Print and shaded views of the part. All mm, measured from the part's lowest x, y and z. A direction names the side the tool comes from. Round coordinates to 2 decimals unless told otherwise and drop trailing zeros. Order: outer loops, then holes, each group sorted by start corner. A loop starts at its lowest first (then second) coordinate and runs counter-clockwise, first axis right, second up. Notation, with made-up numbers: (-3, 11.5) - (6, 11.5) arc R14 cw to (6, 22.5) - close; hole circle Ø9 at (-10, 20.25). An arc over 180 degrees is marked (long way). Write item = value, one per line.
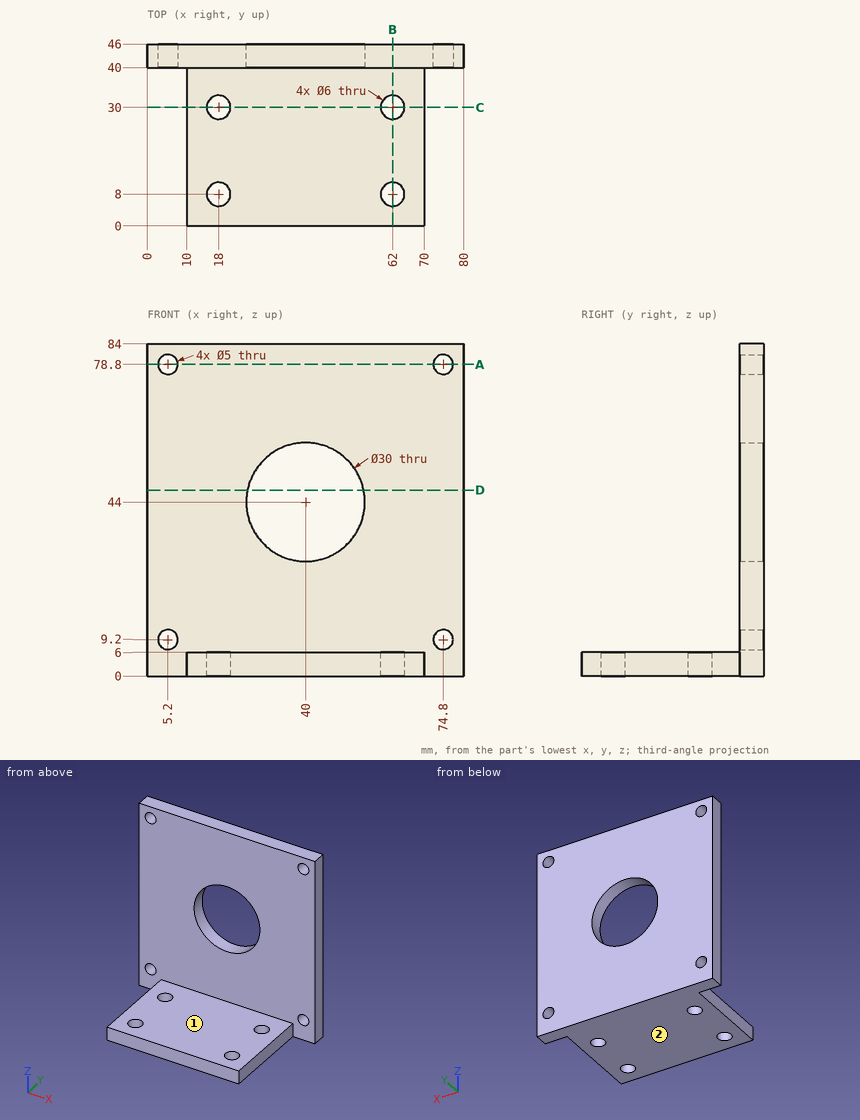
(1) Band-saw the part on B-B on x = 62. List the corners of the cut face in (y, z), plus the area to 3 significant figures.
Solved:
outline = (0, 0) - (5, 0) - (5, 6) - (0, 6) - close; (11, 0) - (27, 0) - (27, 6) - (11, 6) - close; (33, 0) - (46, 0) - (46, 84) - (40, 84) - (40, 6) - (33, 6) - close
area = 672 mm²
(2) Band-saw the part on C-C on y = 30. List the corners of the cut face in (x, z), plus the area to 3 significant figures.
Solved:
outline = (10, 0) - (15, 0) - (15, 6) - (10, 6) - close; (21, 0) - (59, 0) - (59, 6) - (21, 6) - close; (65, 0) - (70, 0) - (70, 6) - (65, 6) - close
area = 288 mm²
(3) Band-saw the part on D-D on z = 47. List the corners of the cut face in (x, y).
Solved:
outline = (0, 40) - (25.3, 40) - (25.3, 46) - (0, 46) - close; (54.7, 40) - (80, 40) - (80, 46) - (54.7, 46) - close
(4) Tool access for the marked faces 1 and 2: list every direction of +Z, -Z, +X, -X, +Y, -Y with a clear straight run to the whole face (end or side of a thin tool).
Solved:
face_1 = +Z, +X, -X, -Y
face_2 = -Z, +X, -X, +Y, -Y
(5) Probe line 1 along Y through (x, z) = (62, 2.75); line 2 along Z through (x, y) = (5.2, 42.6); line 3 along X through (y, z) = (41, 9). List the from-to ranges inside material, lowest first.
Solved:
line_1 = 0 to 5, 11 to 27, 33 to 46
line_2 = 0 to 6.7, 11.7 to 76.3, 81.3 to 84
line_3 = 0 to 2.71, 7.69 to 72.31, 77.29 to 80
(6) Band-saw the part on A-A on z = 78.8. List the corners of the cut face in (x, y), plus the area to 3 significant figures.
Solved:
outline = (0, 40) - (2.7, 40) - (2.7, 46) - (0, 46) - close; (7.7, 40) - (72.3, 40) - (72.3, 46) - (7.7, 46) - close; (77.3, 40) - (80, 40) - (80, 46) - (77.3, 46) - close
area = 420 mm²
(7) Drop flat-ended pins along their axis: pin 1 (6.5 mm diameter, centred on x = 74.8, z = 9.2, fed in from -Y); pin 2 (1.8 mm diameter, centred on y = 25, z = 2, fed in from -X); pin 3 (5 mm diameter, centred on y = 11.5, z = 3.5, fed in from +X). Give the stop position or say it passes through.
Solved:
pin_1 = 40
pin_2 = 10
pin_3 = 70
